The model under review builds one solid part; all positions refer to its coordinate system, in mm. A direction names the side the tool comes from. Round coordinates to 2 decimals unless told otherwise and drop trailing zeros. Write each loop counter-clockwise with the first axis right and the second up, starting at its lowest first coordinate (ties: lowest second). Pieces come first, ordered by that corner, then holes. Notation, with made-up numbers: (-39.75, 58) -> (-22.75, 58) arc R28 ccw to (-22.75, 88) -> close; hole circle Ø8 at (52.25, 76.5). An arc over 180 degrees is marked (long way). Answer in a Markdown table with one row per item. Add a question column.
```python
from build123d import *

# Parameters (mm, degrees)
BOSS_EXTRUDE1_DEPTH = 1.6
SKETCH2_W           = 10.577290559
SKETCH2_H           = 11.232520948
BOSS_EXTRUDE2_DEPTH = 1.6


with BuildPart() as part:
    # Sketch1 → Boss-Extrude1 (new body)
    with BuildSketch(Plane(origin=(0, 0, 0), x_dir=(1, 0, 0), z_dir=(0, 1, 0))):
        with BuildLine():
            Line((-22.9, 11.43), (22.9, 11.43))
            ThreePointArc((22.9, 11.43), (24.667766953, 10.697766953), (25.4, 8.93))
            Line((25.4, 8.93), (25.4, -8.93))
            ThreePointArc((25.4, -8.93), (24.667766953, -10.697766953), (22.9, -11.43))
            Line((22.9, -11.43), (-22.9, -11.43))
            ThreePointArc((-22.9, -11.43), (-24.667766953, -10.697766953), (-25.4, -8.93))
            Line((-25.4, -8.93), (-25.4, 8.93))
            ThreePointArc((-25.4, 8.93), (-24.667766953, 10.697766953), (-22.9, 11.43))
        make_face()
    extrude(amount=BOSS_EXTRUDE1_DEPTH)

    # Sketch2 → Boss-Extrude2 (add)
    with BuildSketch(Plane(origin=(0, 1.6, 0), x_dir=(1, 0, 0), z_dir=(0, 1, 0))):
        with Locations((22.111354721, 0)):
            Rectangle(SKETCH2_W, SKETCH2_H)
    extrude(amount=BOSS_EXTRUDE2_DEPTH)


solid = part.part
```
1. Add section B-B on y = 1.05. Write out the cut boundary in (x, z).
2. For L1, parallel to X at y = 0.6, z = 2; L2, parallel to Z at x = 22, y = 2.5; L3, parallel to Y at x = -17, z = 6.5, list the stretches that pass through material, from the lowest coordinate up.
3. Add section C-C on x = -10. Write out the cut boundary in (y, z).
4. Add section A-A on z = -4.5. Write out the cut boundary in (x, y).
5. Insertion check: pin 1 Ø0.5 at (y, z) = (0.5, 1.5) entering from +X; pin 2 Ø11.5 at (x, z) = (-11.5, -3) entering from +Y; pin 3 Ø1.8 at (x, y) = (21.5, 3) entering from -Z. Each pin has a flat end and moves straight along its axis. Give the tip position at first contact, or say it passes through.
6. Tool access review of faces 1 (the flat face through (25.4, 1, 0)), 2 (the flat face through (22, 2, -5.616)), 3 (the flat face through (22, 2, 5.616)), 4 (the flat face through (16.823, 2, 0)): name each direction out of +Z, -Z, +X, -X, +Y, -Y from which nothing blocks a thin tool from reaching the whole face with its end or side.
Filled in:
| question | item | result |
|---|---|---|
| 1 | outline | (-25.4, -8.93) arc R2.5 ccw to (-22.9, -11.43) -> (22.9, -11.43) arc R2.5 ccw to (25.4, -8.93) -> (25.4, 8.93) arc R2.5 ccw to (22.9, 11.43) -> (-22.9, 11.43) arc R2.5 ccw to (-25.4, 8.93) -> close |
| 2 | L1 | -25.4 to 25.4 |
| 2 | L2 | -5.62 to 5.62 |
| 2 | L3 | 0 to 1.6 |
| 3 | outline | (0, -11.43) -> (1.6, -11.43) -> (1.6, 11.43) -> (0, 11.43) -> close |
| 4 | outline | (-25.4, 0) -> (25.4, 0) -> (25.4, 1.6) -> (27.4, 1.6) -> (27.4, 3.2) -> (16.82, 3.2) -> (16.82, 1.6) -> (-25.4, 1.6) -> close |
| 5 | pin 1 | x = 25.4 |
| 5 | pin 2 | y = 1.6 |
| 5 | pin 3 | z = -5.62 |
| 6 | face 1 | +Z, -Z, +X, -Y |
| 6 | face 2 | -Z, +X, -X, +Y |
| 6 | face 3 | +Z, +X, -X, +Y |
| 6 | face 4 | +Z, -Z, -X, +Y |
